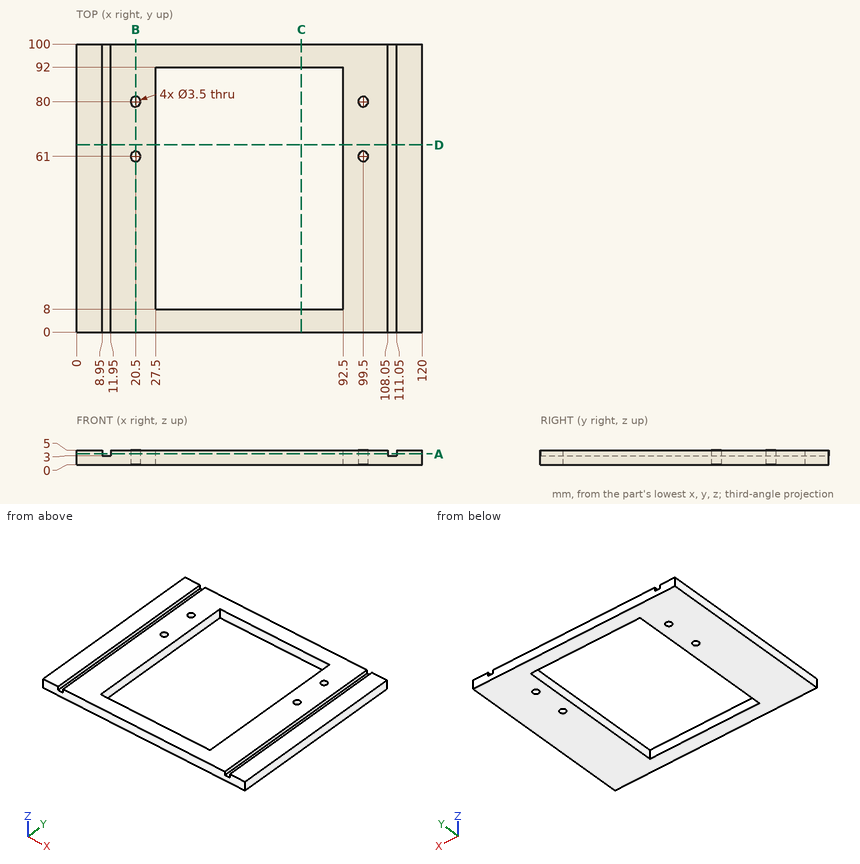
Study the drawing (mm; zero at the part's minimum x, y, z) and answer. Give positions to 0.01 mm unless a question says otherwise; leave off trailing zeros. Write each loop counter-clockwise with the first axis right and the second up, starting at its lowest first coordinate (ties: lowest second). Pieces come first, ordered by that corner, then holes. Notation, with made-up numbers: (-21, 35) - (-8, 35) arc R14 cw to (-8, 42) - close; hole circle Ø2 at (-2, 26.25). An arc over 180 degrees is marked (long way). Write item = value, one per line. Start each with the question number.
Item 1: This flat-tipped pin is pushed along its axis until it touches: P1, Ø0.9, axis at x = 109.5, y = 40, coming from the +Z side. Where does it stop, or does it pass through?
Item 2: Find section A-A (z = 3.75). Give the vertices of the cut face in (x, y).
Item 3: Find the intervals of material crossed by probe 1 along X at (y, z) = (8.5, 4.5); probe 2 along Y at (x, z) = (20.5, 2.4); probe 3 along X at (y, z) = (80, 1.2), in increasing order. Write a range as [from, to].
Item 4: Find section D-D (y = 65). Give the vertices of the cut face in (x, z), then the cut area to 3 significant figures.
Item 5: Find section B-B (x = 20.5). Give the vertices of the cut face in (y, z).
Item 6: Find section C-C (x = 78). Give the vertices of the cut face in (y, z), then the cut area to 3 significant figures.
Response:
q1.P1 = 3
q2.outline = (0, 0) - (8.95, 0) - (8.95, 100) - (0, 100) - close; (11.95, 0) - (108.05, 0) - (108.05, 100) - (11.95, 100) - close; (111.05, 0) - (120, 0) - (120, 100) - (111.05, 100) - close; hole circle Ø3.5 at (20.5, 61); hole circle Ø3.5 at (20.5, 80); hole (27.5, 8) - (92.5, 8) - (92.5, 92) - (27.5, 92) - close; hole circle Ø3.5 at (99.5, 61); hole circle Ø3.5 at (99.5, 80)
q3.probe_1 = [0, 8.95], [11.95, 27.5], [92.5, 108.05], [111.05, 120]
q3.probe_2 = [0, 59.25], [62.75, 78.25], [81.75, 100]
q3.probe_3 = [0, 18.75], [22.25, 27.5], [92.5, 97.75], [101.25, 120]
q4.outline = (0, 0) - (27.5, 0) - (27.5, 5) - (11.95, 5) - (11.95, 3) - (8.95, 3) - (8.95, 5) - (0, 5) - close; (92.5, 0) - (120, 0) - (120, 5) - (111.05, 5) - (111.05, 3) - (108.05, 3) - (108.05, 5) - (92.5, 5) - close
q4.area = 263 mm²
q5.outline = (0, 0) - (59.25, 0) - (59.25, 5) - (0, 5) - close; (62.75, 0) - (78.25, 0) - (78.25, 5) - (62.75, 5) - close; (81.75, 0) - (100, 0) - (100, 5) - (81.75, 5) - close
q6.outline = (0, 0) - (8, 0) - (8, 5) - (0, 5) - close; (92, 0) - (100, 0) - (100, 5) - (92, 5) - close
q6.area = 80.0 mm²
